Can you work these out from the model? Positions are in its coordinate system, mm. A direction names the side the tool comes from. Round coordinates to 2 decimals unless told otherwise and drop trailing zeros. Order: outer loops, then holes, each group sorted by start corner. A loop starts at its lowest first (then second) coordinate and runs counter-clockwise, first axis right, second up. Notation, with made-up numbers: M 87,-33.75 L 113,-33.75 A27 ccw 113,4.25 Z; hole C 20.25,-10 d6. An arc over 180 degrees is marked long. One line per question, with ' | ' between items.
```python
from build123d import *

# Parameters (mm, degrees)
ESQUISSE1_W              = 40
ESQUISSE1_H              = 40
BOSS_EXTRU_1_DEPTH       = 50
ESQUISSE2_R              = 5
ENL_V_MAT_EXTRU_1_DEPTH  = 41
ESQUISSE3_R              = 5
ENL_V_MAT_EXTRU_2_DEPTH  = 41
ESQUISSE4_W              = 22
ESQUISSE4_H              = 14
ENL_V_MAT_EXTRU_3_DEPTH  = 29
ESQUISSE5_W              = 14
ESQUISSE5_H              = 20
ENL_V_MAT_EXTRU_4_DEPTH  = 29
ESQUISSE6_W              = 20
ESQUISSE6_H              = 14
ENL_V_MAT_EXTRU_5_DEPTH  = 24
ESQUISSE7_W              = 14
ESQUISSE7_H              = 22
ENL_V_MAT_EXTRU_6_DEPTH  = 24
ESQUISSE10_R             = 11.25
ENL_V_MAT_EXTRU_9_DEPTH  = 7
ESQUISSE11_R             = 12.75
ENL_V_MAT_EXTRU_10_DEPTH = 1.5
ESQUISSE14_R             = 11.25
ENL_V_MAT_EXTRU_11_DEPTH = 7
ESQUISSE15_R             = 12.75
ENL_V_MAT_EXTRU_12_DEPTH = 1.5
ESQUISSE16_W             = 40
ESQUISSE16_H             = 40
BOSS_EXTRU_2_DEPTH       = 7
ESQUISSE17_R             = 2.25
ENL_V_MAT_EXTRU_13_DEPTH = 15
ESQUISSE18_W             = 3.5
ESQUISSE18_H             = 7.5
ENL_V_MAT_EXTRU_14_DEPTH = 12
ESQUISSE19_W             = 7.5
ESQUISSE19_H             = 3.5
ENL_V_MAT_EXTRU_15_DEPTH = 12


with BuildPart() as part:
    # Esquisse1 → Boss.-Extru.1 (new body)
    with BuildSketch(Plane.XY):
        with Locations((-20, 20)):
            Rectangle(ESQUISSE1_W, ESQUISSE1_H)
    extrude(amount=BOSS_EXTRU_1_DEPTH)

    # Esquisse2 → Enlèv. mat.-Extru.1 (cut, through all)
    with BuildSketch(Plane(origin=(0, 40, 0), x_dir=(1, 0, 0), z_dir=(0, 1, 0))):
        with Locations(Location((-20, -15, 0), (0, 0, 270))):  # turned: the seam where the file's is
            Circle(ESQUISSE2_R)
    extrude(amount=-ENL_V_MAT_EXTRU_1_DEPTH, mode=Mode.SUBTRACT)

    # Esquisse3 → Enlèv. mat.-Extru.2 (cut, through all)
    with BuildSketch(Plane.ZY.offset(40)):
        with Locations((35, 20)):
            Circle(ESQUISSE3_R)
    extrude(amount=-ENL_V_MAT_EXTRU_2_DEPTH, mode=Mode.SUBTRACT)

    # Esquisse4 → Enlèv. mat.-Extru.3 (cut)
    with BuildSketch(Plane.ZY.offset(40)):
        with Locations((11, 20)):
            Rectangle(ESQUISSE4_W, ESQUISSE4_H)
    extrude(amount=-ENL_V_MAT_EXTRU_3_DEPTH, mode=Mode.SUBTRACT)

    # Esquisse5 → Enlèv. mat.-Extru.4 (cut)
    with BuildSketch(Plane.XZ):
        with Locations((-20, 35)):
            Rectangle(ESQUISSE5_W, ESQUISSE5_H)
    extrude(amount=-ENL_V_MAT_EXTRU_4_DEPTH, mode=Mode.SUBTRACT)

    # Esquisse6 → Enlèv. mat.-Extru.5 (cut)
    with BuildSketch(Plane(origin=(0, 0, 0), x_dir=(0, 0, -1), z_dir=(1, 0, 0))):
        with Locations((-15, 20)):
            Rectangle(ESQUISSE6_W, ESQUISSE6_H)
    extrude(amount=-ENL_V_MAT_EXTRU_5_DEPTH, mode=Mode.SUBTRACT)

    # Esquisse7 → Enlèv. mat.-Extru.6 (cut)
    with BuildSketch(Plane(origin=(0, 40, 0), x_dir=(1, 0, 0), z_dir=(0, 1, 0))):
        with Locations((-20, -39)):
            Rectangle(ESQUISSE7_W, ESQUISSE7_H)
    extrude(amount=-ENL_V_MAT_EXTRU_6_DEPTH, mode=Mode.SUBTRACT)

    # Esquisse10 → Enlèv. mat.-Extru.9 (cut)
    with BuildSketch(Plane(origin=(0, 40, 0), x_dir=(1, 0, 0), z_dir=(0, 1, 0))):
        with Locations(Location((-20, -15, 0), (0, 0, 270))):  # turned: the seam where the file's is
            Circle(ESQUISSE10_R)
    extrude(amount=-ENL_V_MAT_EXTRU_9_DEPTH, mode=Mode.SUBTRACT)

    # Esquisse11 → Enlèv. mat.-Extru.10 (cut)
    with BuildSketch(Plane(origin=(0, 40, 0), x_dir=(1, 0, 0), z_dir=(0, 1, 0))):
        with Locations(Location((-20, -15, 0), (0, 0, 270))):  # turned: the seam where the file's is
            Circle(ESQUISSE11_R)
    extrude(amount=-ENL_V_MAT_EXTRU_10_DEPTH, mode=Mode.SUBTRACT)

    # Esquisse14 → Enlèv. mat.-Extru.11 (cut)
    with BuildSketch(Plane.ZY.offset(40)):
        with Locations((35, 20)):
            Circle(ESQUISSE14_R)
    extrude(amount=-ENL_V_MAT_EXTRU_11_DEPTH, mode=Mode.SUBTRACT)

    # Esquisse15 → Enlèv. mat.-Extru.12 (cut)
    with BuildSketch(Plane.ZY.offset(40)):
        with Locations((35, 20)):
            Circle(ESQUISSE15_R)
    extrude(amount=-ENL_V_MAT_EXTRU_12_DEPTH, mode=Mode.SUBTRACT)

    # Esquisse16 → Boss.-Extru.2 (add)
    with BuildSketch(Plane(origin=(0, 0, 0), x_dir=(-1, 0, 0), z_dir=(0, 0, -1))):
        with Locations((20, 20)):
            Rectangle(ESQUISSE16_W, ESQUISSE16_H)
    extrude(amount=BOSS_EXTRU_2_DEPTH)

    # Esquisse17 → Enlèv. mat.-Extru.13 (cut)
    with BuildSketch(Plane(origin=(0, 0, -7), x_dir=(-1, 0, 0), z_dir=(0, 0, -1))):
        with Locations((7.5, 30)):
            Circle(ESQUISSE17_R)
        with Locations((30, 7.5)):
            Circle(ESQUISSE17_R)
    extrude(amount=-ENL_V_MAT_EXTRU_13_DEPTH, mode=Mode.SUBTRACT)

    # Esquisse18 → Enlèv. mat.-Extru.14 (cut)
    with BuildSketch(Plane(origin=(0, 0, 0), x_dir=(0, 0, -1), z_dir=(1, 0, 0))):
        with Locations((1.25, 30)):
            Rectangle(ESQUISSE18_W, ESQUISSE18_H)
    extrude(amount=-ENL_V_MAT_EXTRU_14_DEPTH, mode=Mode.SUBTRACT)

    # Esquisse19 → Enlèv. mat.-Extru.15 (cut)
    with BuildSketch(Plane.XZ):
        with Locations((-30, -1.25)):
            Rectangle(ESQUISSE19_W, ESQUISSE19_H)
    extrude(amount=-ENL_V_MAT_EXTRU_15_DEPTH, mode=Mode.SUBTRACT)


solid = part.part
```
(1) If we section it at C-C on x = -36: Please give me the cut outline in (y, z), plus the area to 3 significant figures.
Final values:
outline: M 0,-7 L 40,-7 L 40,50 L 0,50 Z; hole C 20,35 d22.5; hole M 13,0 L 27,0 L 27,22 L 13,22 Z | area: 1,570 mm^2
(2) Please list where these lines run through material, in increasing order: probe 1 along Z at (x, y) = (-9, 20); probe 2 along Y at (x, z) = (-31.35, 35); probe 3 along X at (y, z) = (39.55, 15). Write a range as [from, to].
Final values:
probe 1: [-7, 5], [25, 30], [40, 50] | probe 2: [0, 15], [25, 40] | probe 3: [-40, -32.75], [-7.25, 0]
(3) On a 3-axis mill with a long thin cutter (end or side, diameter ignored), from which of +Z, -Z, +X, -X, +Y, -Y can I reach the whole of each face in a straight line? I mean faces 4 (the cylindrical face through (-30.982, 35.788, 12.561)), 5 (the flat face through (-20, 29, 27)), 6 (the flat face through (-30, 5, 0.5)). Say none if no direction works.
Final values:
face 4: +Y | face 5: +Z, -Y | face 6: -Y
(4) Will these pins go through, and if not, where does the flat tip stop? pin 1 Ø10 at (y, z) = (35.5, 26) entering from +X; pin 2 Ø1 at (y, z) = (14.5, 39.5) entering from -X; pin 3 Ø3 at (y, z) = (10, 33.5) entering from -X; pin 4 Ø1.8 at (y, z) = (28.5, -2) entering from +X.
Final values:
pin 1: x = 0 | pin 2: x = -33 | pin 3: x = -38.5 | pin 4: x = -12
(5) If we section it at A-A on y = 20: State how many separate pieces and enclosed holes the cut face has, plus the area to 3 significant figures.
Final values:
separate pieces: 5 | enclosed holes: 0 | area: 681 mm^2
(6) If we section it at B-B on z = 15: Please give me the cut outline in (x, y), plus the area to 3 significant figures.
Final values:
outline: M -40,0 L -25,0 L -25,13 L -40,13 Z; M -40,27 L -25,27 L -25,33 L -31.25,33 L -31.25,38.5 L -32.75,38.5 L -32.75,40 L -40,40 Z; M -15,0 L 0,0 L 0,13 L -15,13 Z; M -15,27 L 0,27 L 0,40 L -7.25,40 L -7.25,38.5 L -8.75,38.5 L -8.75,33 L -15,33 Z | area: 688 mm^2
(7) Thinking about a two-plate mould opening in X: for faces 1 (the flat face through (-24, 20, 24)), 2 (the flat face through (-20.3, 15.8, 50)), 3 (the cylindrical face through (-5.252, 30.099, 4.198)), which applies, released by +X, released by -X, zero draft, split by the parting line, or undercut?
Final values:
face 1: released by +X | face 2: zero draft | face 3: undercut
